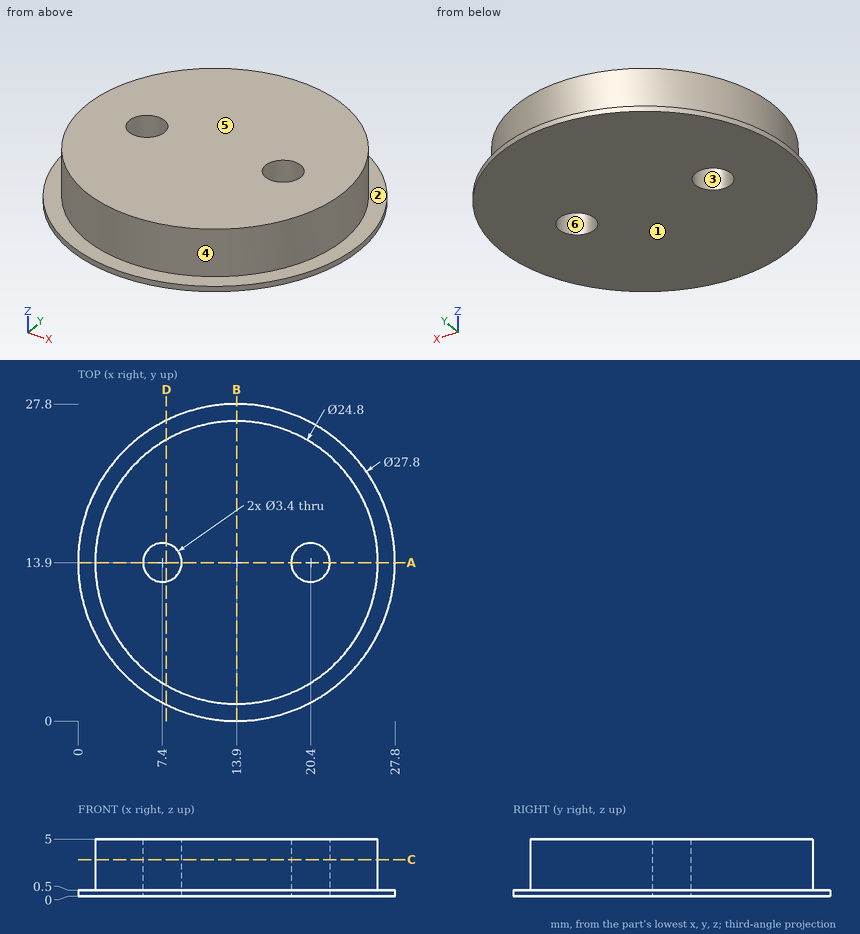
Source: three-view drawing plus pictorial views. Frame: mm from the lowest corner of the part. A direction names the side the tool comes from. Give positions to 0.01 mm unless a question says otherwise; leave off trailing zeros. Loops run counter-clockwise (first coordinate to the right, second up) from the corner with the lowest first, then second, coordinate; pieces in that order, holes last. Notation, with made-up numbers: (24, -1.5) -> (58, -1.5) arc R6 ccw to (58, 9.5) -> close; hole circle Ø6 at (47, 77.5). An arc over 180 degrees is marked (long way). Use a Markdown table: item, result. Add a question column.
(1) Ray query, line 1 (Y direction, x = 7.4, z = 2); line 2 (Y direction, x = 8.5, z = 3.6); line 3 (Y direction, x = 23.75, z = 4.4). Return the intervals inside material, ascending.
(2) First-contact query: pin 1 Ø2 at (y, z) = (18, 4.5) entering from +X; pin 2 Ø8 at (x, y) = (11.5, 8) entering from -Z; pin 3 Ø1.5 at (y, z) = (12, 4) entering from -X; pin 4 Ø1 at (y, z) = (15, 2) entering from -X. Flat tips, straight axial feed; report the tip coordinate or a pass-through.
(3) Section query C-C (z = 3.2). Output: boundary loops of the cut face in (x, y), then the cut area to 3 significant figures.
(4) Section query A-A (y = 13.9). Output: boundary loops of the cut face in (x, z), then the cut area to 3 significant figures.
(5) Section query B-B (x = 13.9). Output: boundary loops of the cut face in (y, z), then the cut area to 4 significant figures.
(6) Pull-direction query (Y, two-part tool) for the marked faces 3, 4, 5 and 6; classes: +Y half, -Y half, draft (parallel to the pull), parting line (faces both ways), or undercut.
(7) Access query for the marked faces 1 and 2. Directions: +Z, -Z, +X, -X, +Y, -Y. A direction counts if a zero-diameter tool reaches every point of the face in a straight line with its end or side. Return the directions, or none.
(8) Section query D-D (x = 7.75). Output: boundary loops of the cut face in (y, z).
Checked values:
| question | item | result |
|---|---|---|
| 1 | line 1 | 3.34 to 12.2, 15.6 to 24.46 |
| 1 | line 2 | 2.74 to 12.6, 15.2 to 25.06 |
| 1 | line 3 | 6.37 to 21.43 |
| 2 | pin 1 | x = 25.91 |
| 2 | pin 2 | z = 0 |
| 2 | pin 3 | x = 1.55 |
| 2 | pin 4 | x = 1.51 |
| 3 | outline | circle Ø24.8 at (13.9, 13.9); hole circle Ø3.4 at (7.4, 13.9); hole circle Ø3.4 at (20.4, 13.9) |
| 3 | area | 465 mm^2 |
| 4 | outline | (0, 0) -> (5.7, 0) -> (5.7, 5) -> (1.5, 5) -> (1.5, 0.5) -> (0, 0.5) -> close; (9.1, 0) -> (18.7, 0) -> (18.7, 5) -> (9.1, 5) -> close; (22.1, 0) -> (27.8, 0) -> (27.8, 0.5) -> (26.3, 0.5) -> (26.3, 5) -> (22.1, 5) -> close |
| 4 | area | 91.5 mm^2 |
| 5 | outline | (0, 0) -> (27.8, 0) -> (27.8, 0.5) -> (26.3, 0.5) -> (26.3, 5) -> (1.5, 5) -> (1.5, 0.5) -> (0, 0.5) -> close |
| 5 | area | 125.5 mm^2 |
| 6 | face 3 | undercut |
| 6 | face 4 | parting line |
| 6 | face 5 | draft |
| 6 | face 6 | undercut |
| 7 | face 1 | -Z, +X, -X, +Y, -Y |
| 7 | face 2 | +Z |
| 8 | outline | (1.43, 0) -> (12.24, 0) -> (12.24, 5) -> (3.13, 5) -> (3.13, 0.5) -> (1.43, 0.5) -> close; (15.56, 0) -> (26.37, 0) -> (26.37, 0.5) -> (24.67, 0.5) -> (24.67, 5) -> (15.56, 5) -> close |
